For this review, use the dimensioned drawing (mm, ordinates from the lowest corner) and the shaded views. A direction names the side the tool comes from. Round coordinates to 2 decimals unless told otherwise and drop trailing zeros. Loops run counter-clockwise (first coordinate to the right, second up) from the corner with the lowest first, then second, coordinate; pieces in that order, holes last. Notation, with made-up numbers: (13, 78.25) - (41, 78.25) arc R28 cw to (41, 106.25) - close; hole circle Ø9 at (-12, 20.25). An arc over 180 degrees is marked (long way). Use one line per item in the form item = value. Start each with the question number.
(1) We need section C-C, the plane x = 41. Write out the cut boundary in (y, z).
(2) Machinability: for the marked faces 4 and 5, which of the approach directions +Z, -Z, +X, -X, +Y, -Y give a long, thin tool a straight path to every point of the face, cutting with its end or side? Answer none if there is none.
(3) We need section D-D, the plane x = 84. Write out the cut boundary in (y, z).
(4) We need section B-B, the plane y = 8.75. Write out the cut boundary in (x, z).
(5) For pin 1 (3.5 mm diameter, centred on x = 84.9, z = 4.9, fed in from +Y); pin 2 (5.5 mm diameter, centred on x = 4.9, z = 4.9, fed in from -Y), all flat-tipped, find the tip position at first contact; note any pin that passes through.
(6) Wall thickness on probe 1 along Z at (x, y) = (48.5, 12.75); probe 2 along Z at (x, y) = (4.5, 1.75) (1 decimal): over which ranges is each line inside the solid? List them lowest first. Write a range as [from, to].
(7) We need section A-A, the plane z = 39.5. Write out the cut boundary in (x, y), then the cut area to 3 significant figures.
(8) The part is to be moulded in two halves that separate along Z. For the marked faces 1, 2 and 3, say which applies: released by +Z, released by -Z, zero draft, split by the parting line, or undercut.
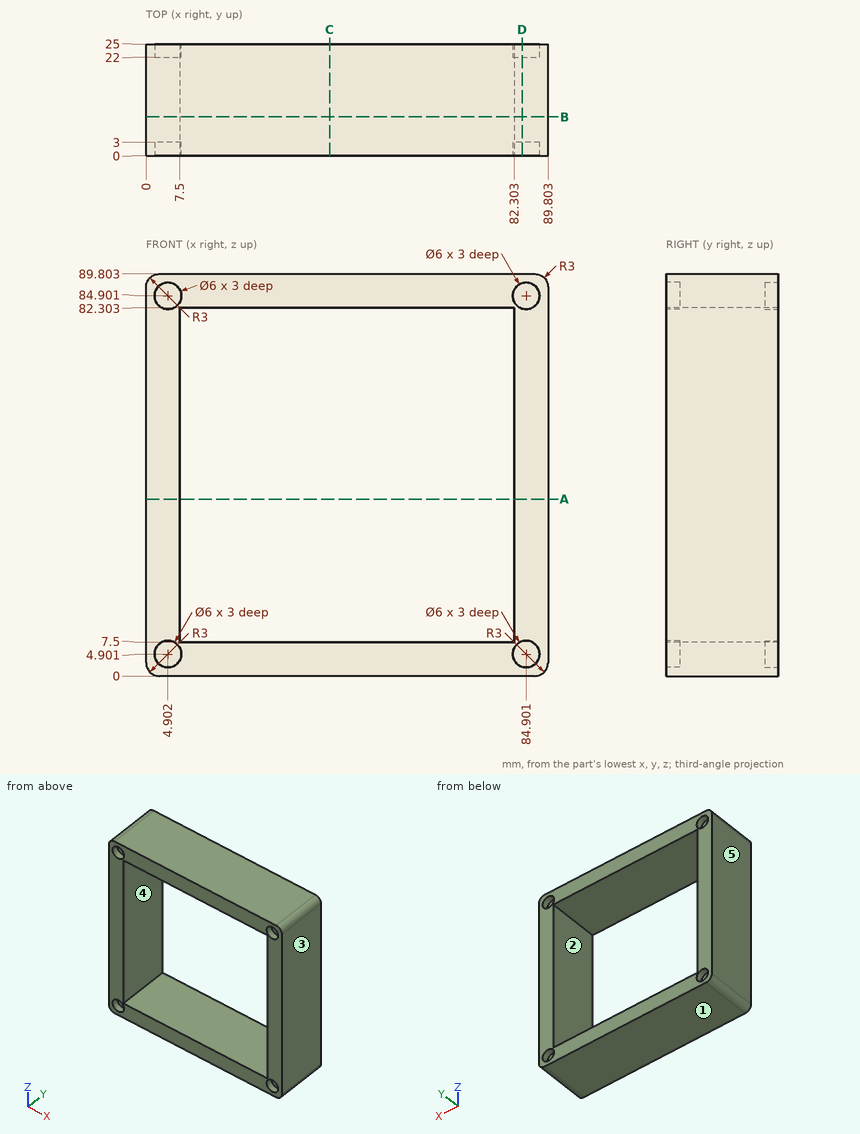
Data:
q1.outline = (0, 0) - (25, 0) - (25, 7.5) - (0, 7.5) - close; (0, 82.3) - (25, 82.3) - (25, 89.8) - (0, 89.8) - close
q2.face_4 = +Y, -Y
q2.face_5 = +Z, -Z, -X, +Y, -Y
q3.outline = (0, 0) - (25, 0) - (25, 2.04) - (22, 2.04) - (22, 7.76) - (25, 7.76) - (25, 82.04) - (22, 82.04) - (22, 87.76) - (25, 87.76) - (25, 89.8) - (0, 89.8) - (0, 87.76) - (3, 87.76) - (3, 82.04) - (0, 82.04) - (0, 7.76) - (3, 7.76) - (3, 2.04) - (0, 2.04) - close
q4.outline = (0, 3) arc R3 ccw to (3, 0) - (86.8, 0) arc R3 ccw to (89.8, 3) - (89.8, 86.8) arc R3 ccw to (86.8, 89.8) - (3, 89.8) arc R3 ccw to (0, 86.8) - close; hole (7.5, 7.5) - (82.3, 7.5) - (82.3, 82.3) - (7.5, 82.3) - close
q5.pin_1 = 22
q5.pin_2 = 3
q6.probe_1 = [0, 7.5], [82.3, 89.8]
q6.probe_2 = [0, 1.9], [7.9, 81.9], [87.9, 89.8]
q7.outline = (0, 0) - (7.5, 0) - (7.5, 25) - (0, 25) - close; (82.3, 0) - (89.8, 0) - (89.8, 25) - (82.3, 25) - close
q7.area = 375 mm^2
q8.face_1 = released by -Z
q8.face_2 = undercut
q8.face_3 = zero draft
